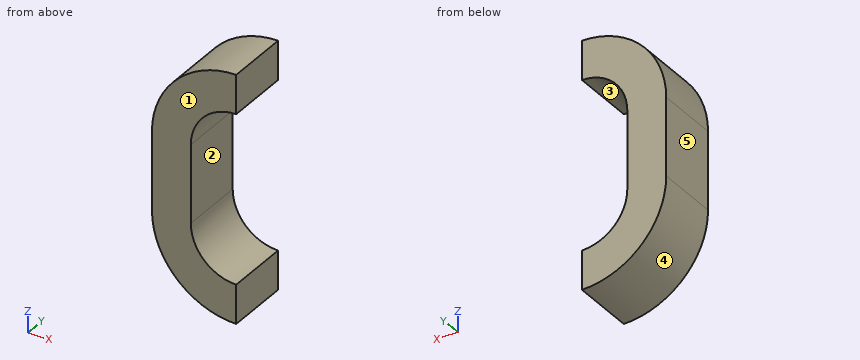
from build123d import *

# Parameters (mm, degrees)
F1_W = 38.1
F1_H = 63.5


with BuildPart() as f2:
    # F2: sweep along a path in F0
    with BuildLine(Plane.XZ) as f2_path:
        Line((-63.5, 0), (-63.5, 38.1))
        ThreePointArc((-63.5, 38.1), (-44.901281, 83.001281), (0, 101.6))
    # F1 (on Top) → F2 (sweep)
    with BuildSketch(Plane.XY):
        with Locations((-63.5, 0)):
            Rectangle(F1_W, F1_H)
    sweep(path=f2_path.line)

    # F3: sweep along a path in F0
    with BuildLine(Plane.XZ) as f3_path:
        Line((-63.5, 0), (-63.5, -38.1))
        ThreePointArc((-63.5, -38.1), (-44.901281, -83.001281), (0, -101.6))
    # F1 (on Top) → F3 (sweep)
    with BuildSketch(Plane.XY):
        with Locations((-63.5, 0)):
            Rectangle(F1_W, F1_H)
    sweep(path=f3_path.line)


solid = f2.part
Work out the finished part from the listing and answer in its coordinate system (mm). Face numbers are marked on the shaded views. A direction names the side the tool comes from. Round coordinates to 2 decimals unless told otherwise and drop trailing zeros. Write each loop counter-clockwise with the first axis right and the second up, starting at its lowest first coordinate (ties: lowest second). Pieces come first, ordered by that corner, then holes. Notation, with made-up numbers: (29.25, 12) - (78.25, 12) arc R19 cw to (78.25, 31) - close; hole circle Ø4 at (-2, 83.5). An arc over 180 degrees is marked (long way). Answer in a Markdown table with one row per item. Add a question column.
1. For the marked faces 1 and 2, determine the directions among +Z, -Z, +X, -X, +Y, -Y from which every point of the face is accessible in a straight line to the end or side of a thin tool.
2. Find the intervals of material crossed by line 1 along X through (y, z) = (-20, 34.5); line 2 along Z through (x, y) = (-25.5, 22); line 3 along Z through (x, y) = (-36, -3), in increasing order. Write a range as from..to.
3. The mould has two halves that part along Z. Classify the marked faces 3, 4 and 5: +Z half, -Z half, draft (parallel to the pull), parting line (faces both ways), or undercut.
4. Given pin 1 (4 mm diameter, centred on x = -62.5, y = -23, fed in from +Z); pin 2 (6 mm diameter, centred on y = 12.5, z = 58.5, fed in from -X); pin 3 (10 mm diameter, centred on x = -56.5, y = -3.5, fed in from -Z), each flat-ended and moving along its own axis, determine where each tip first touches the part or whether it passes through.
5. A cutting plane is placed at D-D, the plane x = -5. Determine the outline of the cut face in (y, z), and give its area (3 significant figures).
6. A cutting plane is placed at B-B, the plane y = -1. Determine the outline of the cut face in (x, z), and give its area (3 significant figures).
7. A cutting plane is placed at A-A, the plane x = -36.5. Determine the outline of the cut face in (y, z).
8. A cutting plane is placed at C-C, the plane z = -4. Determine the outline of the cut face in (x, y), and give its area (3 significant figures).
Worked out:
| question | item | result |
|---|---|---|
| 1 | face 1 | +Z, -Z, +X, -X, -Y |
| 1 | face 2 | +X, +Y, -Y |
| 2 | line 1 | -82.55..-44.45 |
| 2 | line 2 | -116.61..-74.51, 74.51..116.61 |
| 2 | line 3 | -112.39..-64.17, 64.17..112.39 |
| 3 | face 3 | undercut |
| 3 | face 4 | -Z half |
| 3 | face 5 | draft |
| 4 | pin 1 | z = 94.26 |
| 4 | pin 2 | x = -80.7 |
| 4 | pin 3 | z = -102.62 |
| 5 | outline | (-31.75, -120.5) - (31.75, -120.5) - (31.75, -82.27) - (-31.75, -82.27) - close; (-31.75, 82.27) - (31.75, 82.27) - (31.75, 120.5) - (-31.75, 120.5) - close |
| 5 | area | 4,860 mm^2 |
| 6 | outline | (-82.55, -38.1) arc R82.55 ccw to (0, -120.65) - (0, -82.55) arc R44.45 cw to (-44.45, -38.1) - (-44.45, 38.1) arc R44.45 cw to (0, 82.55) - (0, 120.65) arc R82.55 ccw to (-82.55, 38.1) - close |
| 6 | area | 10,500 mm^2 |
| 7 | outline | (-31.75, -112.14) - (31.75, -112.14) - (31.75, -63.47) - (-31.75, -63.47) - close; (-31.75, 63.47) - (31.75, 63.47) - (31.75, 112.14) - (-31.75, 112.14) - close |
| 8 | outline | (-82.55, -31.75) - (-44.45, -31.75) - (-44.45, 31.75) - (-82.55, 31.75) - close |
| 8 | area | 2,420 mm^2 |
